```python
from build123d import *

# Parameters (mm, degrees)
SKETCH1_W           = 93.98
SKETCH1_H           = 76.2
BOSS_EXTRUDE1_DEPTH = 3.175
SKETCH2_W           = 12.7
SKETCH2_H           = 3.175
SKETCH2_W_2         = 17.78
CUT_EXTRUDE1_DEPTH  = 61.578467503
SKETCH3_W           = 3.175
SKETCH3_H           = 25.4
CUT_EXTRUDE2_DEPTH  = 61.578467503
SKETCH4_R           = 1.5
CUT_EXTRUDE3_DEPTH  = 61.578467503


with BuildPart() as part:
    # Sketch1 → Boss-Extrude1 (new body)
    with BuildSketch(Plane.XY):
        Rectangle(SKETCH1_W, SKETCH1_H)
    extrude(amount=BOSS_EXTRUDE1_DEPTH)

    # Sketch2 → Cut-Extrude1 (cut, through all)
    with BuildSketch(Plane.XY.offset(3.175)):
        with Locations((40.64, 36.5125)):
            Rectangle(SKETCH2_W, SKETCH2_H)
        with Locations((-40.64, -36.5125)):
            Rectangle(SKETCH2_W, SKETCH2_H)
        with Locations((0, -36.5125)):
            Rectangle(SKETCH2_W_2, SKETCH2_H)
        with Locations((40.64, -36.5125)):
            Rectangle(SKETCH2_W, SKETCH2_H)
        with Locations((0, 36.5125)):
            Rectangle(SKETCH2_W_2, SKETCH2_H)
        with Locations((-40.64, 36.5125)):
            Rectangle(SKETCH2_W, SKETCH2_H)
    extrude(amount=-CUT_EXTRUDE1_DEPTH, mode=Mode.SUBTRACT)

    # Sketch3 → Cut-Extrude2 (cut, through all)
    with BuildSketch(Plane(origin=(0, 0, 0), x_dir=(-1, 0, 0), z_dir=(0, 0, -1))):
        with Locations((-45.4025, 0)):
            Rectangle(SKETCH3_W, SKETCH3_H)
        with Locations((45.4025, 0)):
            Rectangle(SKETCH3_W, SKETCH3_H)
    extrude(amount=-CUT_EXTRUDE2_DEPTH, mode=Mode.SUBTRACT)

    # Sketch4 → Cut-Extrude3 (cut, through all)
    with BuildSketch(Plane(origin=(0, 0, 0), x_dir=(-1, 0, 0), z_dir=(0, 0, -1))):
        with Locations((-45.4025, 23.8125)):
            Circle(SKETCH4_R)
        with Locations(Location((-45.4025, -23.8125, 0), (0, 0, 180))):
            Circle(SKETCH4_R)
        with Locations((45.4025, -23.8125)):
            Circle(SKETCH4_R)
        with Locations(Location((45.4025, 23.8125, 0), (0, 0, 180))):
            Circle(SKETCH4_R)
    extrude(amount=-CUT_EXTRUDE3_DEPTH, mode=Mode.SUBTRACT)


solid = part.part
```
Here's how the part is built. I have some questions about the finished solid (model axes, mm). A direction names the side the tool comes from. Coordinates: 2 decimals unless noted, no trailing zeros. Write each loop counter-clockwise with the first axis right and the second up, starting at its lowest first coordinate (ties: lowest second). Pieces come first, ordered by that corner, then holes. Notation, with made-up numbers: (17.25, 72.25) -> (42.25, 72.25) arc R15 cw to (42.25, 77.25) -> close; hole circle Ø5 at (49.5, 22.25). An arc over 180 degrees is marked (long way). Use a Markdown table: item, result. Add a question column.
(1) We'd pull the mould along Y, two halves only. Please class faces 6 (the flat face through (41, 34.925, 2)), 7 (the cylindrical face through (44.6, 25.08, 1.57)), 8 (the flat face through (8.89, 36, 2)), 9 (the flat face through (45, 12.7, 2)): +Y half, -Y half, draft (parallel to the pull), parting line (faces both ways), or undercut.
(2) If we section it at B-B, the plane x = -7: Write out the boundary of the cut face in (y, z) (3 decimals).
(3) If we section it at A-A, the plane z = 2.3: State how many separate pieces and enclosed holes the cut face has, and give its area (3 significant figures).
(4) If we section it at C-C, the plane y = 10.5: Write out the boundary of the cut face in (x, z) (3 decimals), and give its area (3 significant figures).
(5) For faces 1 (the flat face through (-34.29, 36, 2)), 2 (the flat face through (0, 34.925, 2)), 3 (the flat face through (34.29, -37, 2)), 4 (the flat face through (-45, -12.7, 2)), 5 (the flat face through (45, -12.7, 2)), which set-ups out of +Z, -Z, +X, -X, +Y, -Y let a thin tool reach every point of the face, with its end or its side?
(6) I'm going to push flat-ended pins straight in: P1, Ø5, axis at x = -45.4, y = 23.81, coming from the -Z side; P2, Ø1.6, axis at x = -45, z = 1.5, coming from the -Y side (3 decimals); P3, Ø1, axis at y = -1.5, z = 2, coming from the -X side (3 decimals); P4, Ø1, axis at y = -36, z = 1, coming from the -X side. Where does each tip first touch, or does it pass through?
(7) Please list where these lines run through material, in increasing order: line 1 (Y direction, x = -35, z = 2.75) (3 decimals); line 2 (X direction, y = 12.5, z = 0.9) (3 decimals); line 3 (X direction, y = 23, z = 2.45).
Outcome:
| question | item | result |
|---|---|---|
| 1 | face 6 | +Y half |
| 1 | face 7 | undercut |
| 1 | face 8 | draft |
| 1 | face 9 | undercut |
| 2 | outline | (-34.925, 0) -> (34.925, 0) -> (34.925, 3.175) -> (-34.925, 3.175) -> close |
| 3 | separate pieces | 1 |
| 3 | enclosed holes | 4 |
| 3 | area | 6,700 mm^2 |
| 4 | outline | (-43.815, 0) -> (43.815, 0) -> (43.815, 3.175) -> (-43.815, 3.175) -> close |
| 4 | area | 278 mm^2 |
| 5 | face 1 | +Z, -Z, -X, +Y |
| 5 | face 2 | +Z, -Z, +Y |
| 5 | face 3 | +Z, -Z, +X, -Y |
| 5 | face 4 | +Z, -Z, -X |
| 5 | face 5 | +Z, -Z, +X |
| 6 | P1 | stops at z = 0 |
| 6 | P2 | stops at y = -34.925 |
| 6 | P3 | stops at x = -43.815 |
| 6 | P4 | stops at x = -34.29 |
| 7 | line 1 | y = -34.925 to 34.925 |
| 7 | line 2 | x = -43.815 to 43.815 |
| 7 | line 3 | x = -46.99 to -46.66, -44.14 to 44.14, 46.66 to 46.99 |
